```python
from build123d import *

# Parameters (mm, degrees)
F0_W       = 20
F0_H       = 25
F0_R       = 2.375
F1_DEPTH   = 2.5
F3_DEPTH   = 10
F4_SIZE2   = 7.49999
F4_SIZE    = 9.99999
F4_2_SIZE2 = 7.49999
F4_2_SIZE  = 9.99999
F5_DEPTH   = 5
F6_R       = 3
F7_DEPTH   = 2.5


# Not quite as in the source:
# - a fillet or chamfer is up to 0.001 mm smaller than in the source, because OpenCascade refuses the exact size


with BuildPart() as f1:
    # F0 (on Top) → F1 (new body)
    with BuildSketch(Plane.XY):
        with Locations((-35.0395915519, -25.5869545043)):
            Rectangle(F0_W, F0_H)
        with Locations((-35.0395915519, -23.0869545043)):
            Circle(F0_R, mode=Mode.SUBTRACT)
    extrude(amount=F1_DEPTH)

    # F2 (on face) → F3 (join)
    with BuildSketch(Plane.XY.offset(2.5)):
        Polygon((-42.5395915519, -28.0869545043), (-45.0395915519, -28.0869545043), (-45.0395915519, -38.0869545043), (-25.0395915519, -38.0869545043), (-25.0395915519, -28.0869545043), (-27.5395915519, -28.0869545043), (-27.5395915519, -35.5869545043), (-42.5395915519, -35.5869545043), align=None)
    extrude(amount=F3_DEPTH)

    # F4 (size 10 and 7.5 in the source; OpenCascade refuses exactly that, so slightly less here)
    f4_edges = [f1.edges().sort_by_distance(p)[0] for p in [
        (-43.789592, -28.086955, 12.5),
    ]]
    f4_side = f1.faces().sort_by_distance((-43.789592, -28.086955, 7.5))[0]
    chamfer(f4_edges, length=F4_SIZE, length2=F4_SIZE2, reference=f4_side)

    # F4#2 (size 10 and 7.5 in the source; OpenCascade refuses exactly that, so slightly less here)
    f4_2_edges = [f1.edges().sort_by_distance(p)[0] for p in [
        (-26.289592, -28.086955, 12.5),
    ]]
    f4_2_side = f1.faces().sort_by_distance((-26.289592, -28.086955, 7.5))[0]
    chamfer(f4_2_edges, length=F4_2_SIZE, length2=F4_2_SIZE2, reference=f4_2_side)

    # F5 (add): a face of the model
    f5_faces = [f1.faces().sort_by_distance(p)[0] for p in [
        (-35.0395915519, -36.8369532542, 12.5),
    ]]
    extrude(f5_faces, amount=F5_DEPTH)

    # F6 (on face) → F7 (cut)
    with BuildSketch(Plane.XZ.offset(38.0869545043)):
        with Locations((-35.0395915519, 7.25)):
            Circle(F6_R)
    extrude(amount=-F7_DEPTH, mode=Mode.SUBTRACT)


solid = f1.part
```
Work out the finished part from the listing and answer in its coordinate system (mm). A direction names the side the tool comes from. Give positions to 0.01 mm unless a question says otherwise; leave off trailing zeros. Loops run counter-clockwise (first coordinate to the right, second up) from the corner with the lowest first, then second, coordinate; pieces in that order, holes last. Notation, with made-up numbers: (-29, -33.5) -> (-1, -33.5) arc R29 ccw to (-1, -2.5) -> close; hole circle Ø8 at (80.5, 59). An arc over 180 degrees is marked (long way). Put each result on its own line as item: value. Start each with the question number.
Item 1: The part is cut by section D-D (y = -27.5). Give the vertices of the cut face in (x, z), then the cut area to 3 significant figures.
Item 2: Find the intervals of material crossed by L1, parallel to X at y = -30.25, z = 3.5; L2, parallel to Z at x = -37.75, y = -16; L3, parallel to Y at x = -33, z = 5, in increasing order. Write a range as [from, to].
Item 3: The mould has two halves that part along X. Classify faces 4 (the face through (-45.04, -30, 4)), 5 (the face through (-37, -25, 0)), 6 (the face through (-27.54, -33, 6)): released by +X, released by -X, zero draft, split by the parting line, or undercut.
Item 4: The part is cut by section B-B (x = -38.5). Give the vertices of the cut face in (y, z).
Item 5: Which of the six approach directions +Z, -Z, +X, -X, +Y, -Y give full straight-line access (tool end or side, diameter ignored) to faces 1 (the face through (-35, -37, 17.5)), 2 (the face through (-26, -35.587, 15)), 3 (the face through (-35, -35.587, 12))?
Item 6: The part is cut by section C-C (z = 16.75). Give the vertices of the cut face in (x, y), then the cut area to 3 significant figures.
Item 7: Each of these flat-tipped pins is pushed along its axis until it touches: P1, Ø12, axis at x = -33, y = -24, coming from the +Z side; P2, Ø1.2, axis at x = -27, z = 14.5, coming from the +Y side; P3, Ø5, axis at x = -35.04, z = 7.25, coming from the +Y side. Where does it stop, or does it pass through?
Item 8: The part is cut by section A-A (z = 6.75). Give the vertices of the cut face in (x, y).
Answers below:
1. outline: (-45.04, 0) -> (-25.04, 0) -> (-25.04, 2.5) -> (-45.04, 2.5) -> close
1. area: 50.0 mm2
2. L1: [-45.04, -42.54], [-27.54, -25.04]
2. L2: [0, 2.5]
2. L3: [-38.09, -35.59]
3. face 4: released by -X
3. face 5: zero draft
3. face 6: undercut
4. outline: (-38.09, 0) -> (-13.09, 0) -> (-13.09, 2.5) -> (-35.59, 2.5) -> (-35.59, 17.5) -> (-38.09, 17.5) -> close
5. face 1: +Z, +X, -X, +Y, -Y
5. face 2: +Z, +X, -X, +Y
5. face 3: +Z, +Y
6. outline: (-45.04, -38.09) -> (-25.04, -38.09) -> (-25.04, -35.59) -> (-42.54, -35.59) -> (-45.04, -35.59) -> close
6. area: 50.0 mm2
7. P1: z = 2.5
7. P2: y = -35.59
7. P3: through
8. outline: (-45.04, -38.09) -> (-38, -38.09) -> (-38, -35.59) -> (-42.54, -35.59) -> (-42.54, -31.27) -> (-45.04, -31.27) -> close; (-32.08, -38.09) -> (-25.04, -38.09) -> (-25.04, -31.27) -> (-27.54, -31.27) -> (-27.54, -35.59) -> (-32.08, -35.59) -> close
